Work out the finished part from the listing and answer in its coordinate system (mm). A direction names the side the tool comes from. Coordinates: 2 decimals unless noted, no trailing zeros. Write each loop counter-clockwise with the first axis right and the second up, starting at its lowest first coordinate (ties: lowest second). Pieces come first, ordered by that corner, then holes. Notation, with made-up numbers: (31, 53) - (47, 53) arc R21 cw to (47, 88) - close; hole circle Ø3 at (63, 87.25). An arc over 180 degrees is marked (long way). One line per item, written item: value.
```python
from build123d import *

# Parameters (mm, degrees)
SKETCH1_W           = 6.35
SKETCH1_H           = 203.2
SKETCH1_W_2         = 4.7625
SKETCH1_H_2         = 29.028571429
BOSS_EXTRUDE1_DEPTH = 4.7625


with BuildPart() as part:
    # Sketch1 → Boss-Extrude1 (new body)
    with BuildSketch(Plane.XY):
        with Locations((-3.175, 0)):
            Rectangle(SKETCH1_W, SKETCH1_H)
        Polygon((6.35, 101.6), (0, 101.6), (0, -101.6), (6.35, -101.6), (6.35, -72.571428571), (6.35, -43.542857143), (6.35, -14.514285714), (6.35, 14.514285714), (6.35, 43.542857143), (6.35, 72.571428571), align=None)
        with Locations((8.73125, 87.085714286)):
            Rectangle(SKETCH1_W_2, SKETCH1_H_2)
        with Locations((8.73125, 29.028571429)):
            Rectangle(SKETCH1_W_2, SKETCH1_H_2)
        with Locations((8.73125, -29.028571429)):
            Rectangle(SKETCH1_W_2, SKETCH1_H_2)
        with Locations((8.73125, -87.085714286)):
            Rectangle(SKETCH1_W_2, SKETCH1_H_2)
    extrude(amount=BOSS_EXTRUDE1_DEPTH)


solid = part.part
```
Item 1: Section A-A, the plane z = 3.2 is taken. Determine the outline of the cut face in (x, y).
Evaluation:
outline: (-6.35, -101.6) - (11.11, -101.6) - (11.11, -72.57) - (6.35, -72.57) - (6.35, -43.54) - (11.11, -43.54) - (11.11, -14.51) - (6.35, -14.51) - (6.35, 14.51) - (11.11, 14.51) - (11.11, 43.54) - (6.35, 43.54) - (6.35, 72.57) - (11.11, 72.57) - (11.11, 101.6) - (-6.35, 101.6) - close
Item 2: Consider probe 1 along Y at (x, z) = (9.5, 1.05); probe 2 along X at (y, z) = (64, 1.25). Determine where each line is inside the solid, lowest interval first.
Evaluation:
probe 1: y = -101.6 to -72.57, -43.54 to -14.51, 14.51 to 43.54, 72.57 to 101.6
probe 2: x = -6.35 to 6.35
Item 3: Which of the six approach directions +Z, -Z, +X, -X, +Y, -Y give full straight-line access (tool end or side, diameter ignored) to faces 5 (the face through (11.112, -87, 2)), 6 (the face through (9, -14.514, 2))?
Evaluation:
face 5: +Z, -Z, +X, +Y, -Y
face 6: +Z, -Z, +X
Item 4: Given pin 1 (1.4 mm diameter, centred on y = 63.5, z = 1.5, fed in from +X); pin 2 (2 mm diameter, centred on x = 6.5, y = 57.5, fed in from +Z), each flat-ended and moving along its own axis, determine where each tip first touches the part or whether it passes through.
Evaluation:
pin 1: stops at x = 6.35
pin 2: stops at z = 4.76
Item 5: Determine the mould class of faces 1 (the face through (11.112, 29, 2)), 2 (the face through (2, -101.6, 2)), 3 (the face through (9, -72.571, 2)), 4 (the face through (9, -43.543, 2)) for opening direction Y: +Y half, -Y half, draft (parallel to the pull), parting line (faces both ways), or undercut.
Evaluation:
face 1: draft
face 2: -Y half
face 3: undercut
face 4: undercut
Item 6: Section B-B, the plane y = -68 is taken. Determine the outline of the cut face in (x, z).
Evaluation:
outline: (-6.35, 0) - (6.35, 0) - (6.35, 4.76) - (-6.35, 4.76) - close
